Geometry: final body of the model. Coordinates: model frame, mm. Give positions to 0.01 mm unless a question says otherwise; leave off trailing zeros. Write each loop counter-clockwise with the first axis right and the second up, starting at its lowest first coordinate (ties: lowest second). Pieces come first, ordered by that corner, then holes. Notation, with made-up numbers: (-27, 41.5) -> (14, 41.5) arc R5 ccw to (14, 49.5) -> close; hole circle Ø9 at (80, 5.25). An arc over 180 degrees is marked (long way). Answer in a Markdown table with one row per item. Add a question column.
Item 1: Section query B-B on z = 15. Output: boundary loops of the cut face in (x, y) (3 decimals), plus the area to 3 significant figures.
Item 2: Section query C-C on y = 1.7. Output: boundary loops of the cut face in (x, z) (3 decimals).
Item 3: Section query A-A on x = -13. Output: boundary loops of the cut face in (y, z) (3 decimals), plus the area to 3 significant figures.
Item 4: Material intervals for probe 1 along X at (y, z) = (2.65, -18.5); probe 2 along Z at (x, y) = (55.5, 2.05), sorted ascending. Write a range as from..to.
Autodesk Inventor part; units mm, degrees
ref_plane "YZ Plane" through (0, 0, 0) normal (1, 0, 0) x (0, 1, 0)
ref_plane "XZ Plane" through (0, 0, 0) normal (0, 1, 0) x (-1, 0, 0)
ref_plane "XY Plane" through (0, 0, 0) normal (0, 0, 1) x (1, 0, 0)
sketch "Sketch1" plane through (0, 0, 0) normal (0, 1, 0) x (-1, 0, 0)
  line L0 (-63.5, 63.5) -> (63.5, 63.5)
  line L1 (63.5, 63.5) -> (63.5, -63.5)
  line L2 (63.5, -63.5) -> (-63.5, -63.5)
  line L3 (-63.5, -63.5) -> (-63.5, 63.5)
  line L4 (-50.8, 50.8) -> (50.8, 50.8)
  line L5 (50.8, 50.8) -> (50.8, -50.8)
  line L6 (50.8, -50.8) -> (-50.8, -50.8)
  line L7 (-50.8, -50.8) -> (-50.8, 50.8)
  point P0 (0, 0)
  dimension "d0" = 127
  dimension "d1" = 127
  dimension "d2" = 63.5
  dimension "d3" = 63.5
  dimension "d4" = 50.8
  dimension "d5" = 50.8
  dimension "d6" = 101.6
  dimension "d7" = 101.6
extrude "Extrusion1" add sketch "Sketch1" along normal blind 3.175
fillet "Fillet1" radius 12.7 4 edges at (-50.8, 1.5875, -50.8) (-50.8, 1.5875, 50.8) (50.8, 1.5875, -50.8) (50.8, 1.5875, 50.8)
sketch "Sketch2" plane through (0, 3.175, 0) normal (0, 1, 0) x (1, 0, 0)
  line L0 (63.5, 63.5) -> (-63.5, 63.5)
  line L1 (-63.5, 63.5) -> (-63.5, -63.5)
  circle A0 centre (-53.975, 53.975) radius 3.175
  circle A1 centre (53.975, 53.975) radius 3.175
  circle A2 centre (-53.975, -53.975) radius 3.175
  circle A3 centre (53.975, -53.975) radius 3.175
  point P0 (0, 0)
  dimension "d11" = 6.35
  dimension "d12" = 9.525
  dimension "d13" = 9.525
  dimension "d16" = 107.95
  dimension "d19" = 107.95
extrude "Extrusion2" cut sketch "Sketch2" against normal blind 3.175
properties part number "case1_space"
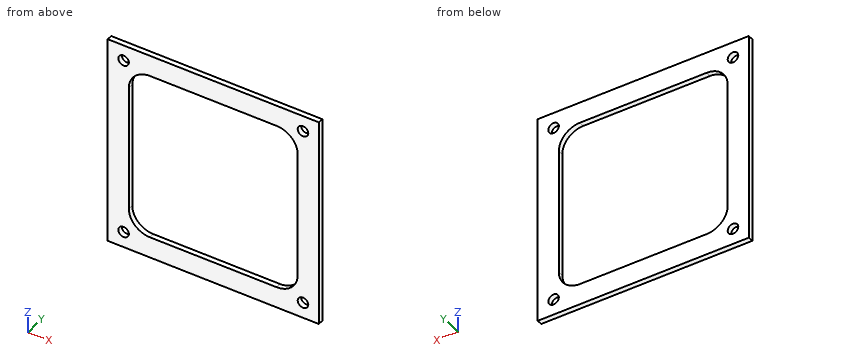
Findings below:
| question | item | result |
|---|---|---|
| 1 | outline | (-63.5, 0) -> (-50.8, 0) -> (-50.8, 3.175) -> (-63.5, 3.175) -> close; (50.8, 0) -> (63.5, 0) -> (63.5, 3.175) -> (50.8, 3.175) -> close |
| 1 | area | 80.6 mm^2 |
| 2 | outline | (-63.5, -63.5) -> (63.5, -63.5) -> (63.5, 63.5) -> (-63.5, 63.5) -> close; hole circle Ø6.35 at (-53.975, -53.975); hole circle Ø6.35 at (-53.975, 53.975); hole (-50.8, -38.1) arc R12.7 ccw to (-38.1, -50.8) -> (38.1, -50.8) arc R12.7 ccw to (50.8, -38.1) -> (50.8, 38.1) arc R12.7 ccw to (38.1, 50.8) -> (-38.1, 50.8) arc R12.7 ccw to (-50.8, 38.1) -> close; hole circle Ø6.35 at (53.975, -53.975); hole circle Ø6.35 at (53.975, 53.975) |
| 3 | outline | (0, -63.5) -> (3.175, -63.5) -> (3.175, -50.8) -> (0, -50.8) -> close; (0, 50.8) -> (3.175, 50.8) -> (3.175, 63.5) -> (0, 63.5) -> close |
| 3 | area | 80.6 mm^2 |
| 4 | probe 1 | x = -63.5..-50.8, 50.8..63.5 |
| 4 | probe 2 | z = -63.5..-56.76, -51.19..51.19, 56.76..63.5 |
